from build123d import *

# Parameters (mm, degrees)
SKETCH1_W           = 42
SKETCH1_H           = 25
BOSS_EXTRUDE1_DEPTH = 2
SKETCH2_W           = 2
SKETCH2_H           = 25
BOSS_EXTRUDE2_DEPTH = 25
SKETCH3_W           = 10
SKETCH3_H           = 1.2
BOSS_EXTRUDE3_DEPTH = 6
FILLET1_R           = 4


with BuildPart() as part:
    # Sketch1 → Boss-Extrude1 (new body)
    with BuildSketch(Plane.XY):
        with Locations((-21, 12.5)):
            Rectangle(SKETCH1_W, SKETCH1_H)
    extrude(amount=BOSS_EXTRUDE1_DEPTH)

    # Sketch2 → Boss-Extrude2 (add)
    with BuildSketch(Plane.XY.offset(2)):
        with Locations((-1, 12.5)):
            Rectangle(SKETCH2_W, SKETCH2_H)
    extrude(amount=BOSS_EXTRUDE2_DEPTH)

    # Sketch3 → Boss-Extrude3 (add)
    with BuildSketch(Plane(origin=(0, 0, 0), x_dir=(0, 0, -1), z_dir=(1, 0, 0))):
        with Locations((-5, 19.4)):
            Rectangle(SKETCH3_W, SKETCH3_H)
        with Locations((-5, 5.6)):
            Rectangle(SKETCH3_W, SKETCH3_H)
    extrude(amount=BOSS_EXTRUDE3_DEPTH)

    # Fillet1
    fillet1_edges = [part.edges().sort_by_distance(p)[0] for p in [
        (-2, 12.5, 2),
    ]]
    fillet(fillet1_edges, radius=FILLET1_R)


solid = part.part
Verification items for the finished model (mm, model axes). A direction names the side the tool comes from. Round coordinates to 2 decimals unless told otherwise and drop trailing zeros. Loops run counter-clockwise (first coordinate to the right, second up) from the corner with the lowest first, then second, coordinate; pieces in that order, holes last. Notation, with made-up numbers: (84, -30) - (125, -30) arc R23 cw to (125, -17) - close; hole circle Ø9 at (-24.5, 65). An arc over 180 degrees is marked (long way). Use one line per item in the form item = value.
1. Gauge pin test, flat ends, axial feed: pin 1 Ø0.6 at (x, y) = (2.5, 19.5) entering from +Z; pin 2 Ø3 at (y, z) = (20.5, 15.5) entering from +X; pin 3 Ø3 at (y, z) = (11, 17.5) entering from -X. Record the tip position at first contact, or that the pin passes through.
A:
pin_1 = 10
pin_2 = 0
pin_3 = -2
2. Section check A-A on z = 8.75. Record the cut outline in (x, y), and give its area (3 significant figures).
A:
outline = (-2, 0) - (0, 0) - (0, 5) - (6, 5) - (6, 6.2) - (0, 6.2) - (0, 18.8) - (6, 18.8) - (6, 20) - (0, 20) - (0, 25) - (-2, 25) - close
area = 64.4 mm²
3. Section check C-C on x = -14.5. Record the cut outline in (y, z).
A:
outline = (0, 0) - (25, 0) - (25, 2) - (0, 2) - close
4. Access from +Z, -Z, +X, -X, +Y, -Y to the whole of each face (thin tool, end or side, straight path). Record for faces 1 (the flat face through (3, 5, 5)), 2 (the flat face through (-24, 13, 2)), 3 (the flat face through (3, 6.2, 5)), 4 (the flat face through (3, 6, 10)), 5 (the flat face through (-15, 25, 1)).
A:
face_1 = +Z, -Z, +X, -Y
face_2 = +Z, -X, +Y, -Y
face_3 = +Z, -Z, +X
face_4 = +Z, +X, +Y, -Y
face_5 = +Z, -Z, +X, -X, +Y
5. Scan lines: probe 1 along Z at (x, y) = (-25.5, 19); probe 2 along X at (y, z) = (4, 16); probe 3 along X at (y, z) = (21.75, 3.75). Record each from-to range of solid material in increasing order.
A:
probe_1 = 0 to 2
probe_2 = -2 to 0
probe_3 = -2.69 to 0
6. Section check D-D on z = 5.5. Record the cut outline in (x, y), and give its area (3 significant figures).
A:
outline = (-2.03, 0) - (0, 0) - (0, 5) - (6, 5) - (6, 6.2) - (0, 6.2) - (0, 18.8) - (6, 18.8) - (6, 20) - (0, 20) - (0, 25) - (-2.03, 25) - close
area = 65.2 mm²
7. Draft check along Y on faces 6 (the flat face through (3, 20, 5)), 7 (the flat face through (-2, 12, 16)), 8 (the flat face through (0, 12, 13)). Enter one of: pulls with the +Y half, pulls with the -Y half, needs draft (parallel to the pull), parting line crosses it, or undercut.
A:
face_6 = pulls with the +Y half
face_7 = needs draft
face_8 = undercut
8. Section check B-B on y = 12. Record the cut outline in (x, z).
A:
outline = (-42, 0) - (0, 0) - (0, 27) - (-2, 27) - (-2, 6) arc R4 cw to (-6, 2) - (-42, 2) - close
